```python
from build123d import *

# Parameters (mm, degrees)
F0_W      = 60
F0_H      = 40
F1_DEPTH  = 50
F2_W      = 10
F2_H      = 35
F4_W      = 10
F4_H      = 10
F10_DEPTH = 50.001
F11_W     = 15
F11_H     = 20
F12_DEPTH = 50.001
F7_W      = 40
F7_H      = 20
F14_W     = 10
F14_H     = 10
F15_DEPTH = 60.001
F14_W_2   = 20
F19_DEPTH = 60.001


with BuildPart() as f1:
    # F0 (on Top) → F1 (new body)
    with BuildSketch(Plane.XY):
        with Locations((30, 20)):
            Rectangle(F0_W, F0_H)
    extrude(amount=F1_DEPTH)

    # F2 (on face) → F3 (revolve, cut)
    with BuildSketch(Plane.XY.offset(50)):
        with Locations((15, 17.5)):
            Rectangle(F2_W, F2_H)
    revolve(axis=Axis((15, 0, 50), (1, 0, 0)), mode=Mode.SUBTRACT)

    # F6: sweep along a path in F5
    with BuildLine(Plane(origin=(0, 0, 0), x_dir=(0, -1, 0), z_dir=(-1, 0, 0))) as f6_path:
        Line((0, 40), (-20, 50))
    # F4 (on face) → F6 (sweep, cut)
    with BuildSketch(Plane.XZ):
        with Locations((5, 45)):
            Rectangle(F4_W, F4_H)
    sweep(path=f6_path.line, mode=Mode.SUBTRACT)

    # F9 (on face) → F10 (cut, through all)
    with BuildSketch(Plane.XY.offset(50)):
        Polygon((45, 20), (30, 0), (45, 0), align=None)
    extrude(amount=-F10_DEPTH, mode=Mode.SUBTRACT)

    # F11 (on face) → F12 (cut, through all)
    with BuildSketch(Plane.XY.offset(50)):
        with Locations((52.5, 10)):
            Rectangle(F11_W, F11_H)
    extrude(amount=-F12_DEPTH, mode=Mode.SUBTRACT)

    # F13: sweep along a path in F8
    with BuildLine(Plane.YZ.offset(60)) as f13_path:
        Line((0, 30), (20, 50))
    # F7 (on face) → F13 (sweep, cut)
    with BuildSketch(Plane.XZ):
        with Locations((40, 40)):
            Rectangle(F7_W, F7_H)
    sweep(path=f13_path.line, mode=Mode.SUBTRACT)

    # F14 (on face) → F15 (cut, through all)
    with BuildSketch(Plane.YZ.offset(60)):
        with Locations((25, 5)):
            Rectangle(F14_W, F14_H)
        with Locations((15, 5)):
            Rectangle(F14_W, F14_H)
    extrude(amount=-F15_DEPTH, mode=Mode.SUBTRACT)

    # F18: sweep along a path in F17
    with BuildLine(Plane.YZ.offset(60)) as f18_path:
        Line((30, 10), (20, 50))
    # F16 (on face) → F18 (sweep, cut)
    with BuildSketch(Plane(origin=(0, 0, 10), x_dir=(1, 0, 0), z_dir=(0, 0, -1))):
        Polygon((60, -20), (45, -20), (60, -30), align=None)
    sweep(path=f18_path.line, mode=Mode.SUBTRACT)

    # F14 (on face) → F19 (cut, through all)
    with BuildSketch(Plane.YZ.offset(60)):
        with Locations((20, 5)):
            Rectangle(F14_W_2, F14_H)
        with Locations((15, 5)):
            Rectangle(F14_W, F14_H)
    extrude(amount=-F19_DEPTH, mode=Mode.SUBTRACT)


solid = f1.part
```
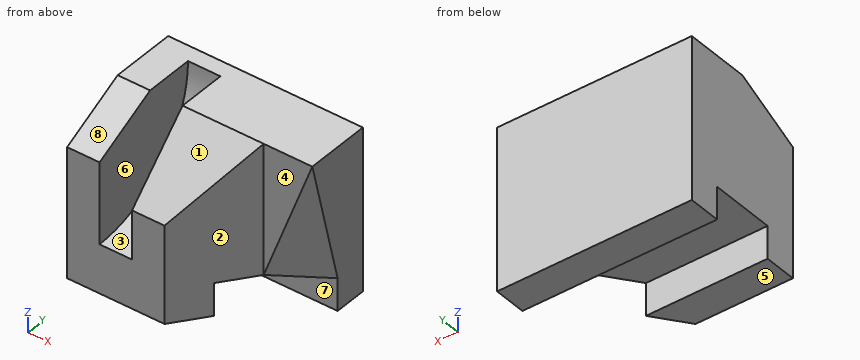
Geometry: final body of the model. Coordinates: model frame, mm. Face numbers are marked on the shaded views. A direction names the side the tool comes from. Coordinates: 2 decimals unless noted, no trailing zeros. Loops run counter-clockwise (first coordinate to the right, second up) from the corner with the lowest first, then second, coordinate; pieces in that order, holes last. Notation, with made-up numbers: (66.25, -25.75) -> (125.25, -25.75) arc R14 ccw to (125.25, -8.75) -> close; hole circle Ø5 at (-21, -0.5). An arc over 180 degrees is marked (long way). Use a Markdown table: item, result. Add a question column.
(1) Access query for the marked faces 4, 5, 6, 7 and 8. Directions: +Z, -Z, +X, -X, +Y, -Y. A direction counts if a zero-diameter tool reaches every point of the face in a straight line with its end or side. Return the directions, or none.
(2) Section query A-A, the plane z = 5.5. Return loops of the section in (x, y), plus the area to 4 significant figures.
(3) Section query D-D, the plane z = 44.5. Return loops of the section in (x, y) (1 decimal), plus the area to 3 significant figures.
(4) Line query: line 1 along Y through (x, z) = (3.5, 6.5); line 2 along X through (y, z) = (17, 33.5); line 3 along X through (y, z) = (12, 43). Output: solid intervals per line, ascending.
(5) Pin query (flat end, axial travel): pin 1 Ø1.5 at (y, z) = (21, 34) entering from +X; pin 2 Ø1.5 at (x, z) = (33, 35) entering from -Y; pin 3 Ø8 at (y, z) = (9, 41.5) entering from +X. Return the tip coordinate at first contact, or that it passes through.
(6) Mould query, pull axis X, two halves, no side actions, for the marked faces 1, 2 and 3. Classes: pulls with the +X half, pulls with the -X half, needs draft (parallel to the pull), parting line crosses it, or undercut.
(7) Section query B-B, the plane x = 27.5. Return loops of the section in (y, z), plus the area to 3 significant figures.
(8) Section query C-C, the plane y = 6. Return loops of the section in (x, z).
Answer:
| question | item | result |
|---|---|---|
| 1 | face 4 | +Z, -Z, +X, -Y |
| 1 | face 5 | -Z, +X, -X, +Y, -Y |
| 1 | face 6 | +Z, -Y |
| 1 | face 7 | -Z, +X, -X |
| 1 | face 8 | +Z, +X, -X, -Y |
| 2 | outline | (0, 0) -> (30, 0) -> (37.5, 10) -> (0, 10) -> close; (0, 30) -> (60, 30) -> (60, 40) -> (0, 40) -> close |
| 2 | area | 937.5 mm^2 |
| 3 | outline | (0, 9) -> (10, 9) -> (10, 34.6) -> (20, 34.6) -> (20, 14.5) -> (40.9, 14.5) -> (45, 20) -> (57.9, 20) -> (60, 21.4) -> (60, 40) -> (0, 40) -> close |
| 3 | area | 1,290 mm^2 |
| 4 | line 1 | y = 0 to 10, 30 to 40 |
| 4 | line 2 | x = 0 to 10, 20 to 42.75 |
| 4 | line 3 | x = 0 to 10 |
| 5 | pin 1 | stops at x = 56.66 |
| 5 | pin 2 | stops at y = 4.25 |
| 5 | pin 3 | stops at x = 39.75 |
| 6 | face 1 | needs draft |
| 6 | face 2 | pulls with the +X half |
| 6 | face 3 | undercut |
| 7 | outline | (0, 0) -> (10, 0) -> (10, 10) -> (30, 10) -> (30, 0) -> (40, 0) -> (40, 50) -> (20, 50) -> (0, 30) -> close |
| 7 | area | 1,600 mm^2 |
| 8 | outline | (0, 0) -> (34.5, 0) -> (34.5, 36) -> (20, 36) -> (20, 15.52) -> (10, 15.52) -> (10, 43) -> (0, 43) -> close |
